from build123d import *

# Parameters (mm, degrees)
SKETCH1_R           = 45.5
SKETCH1_R_2         = 29.5
BOSS_EXTRUDE1_DEPTH = 4
SKETCH2_R           = 37.5
SKETCH2_R_2         = 29.5
BOSS_EXTRUDE2_DEPTH = 79.3
SKETCH4_R           = 1.55
CUT_EXTRUDE1_DEPTH  = 83.3
CIRPATTERN1_COUNT   = 3
SKETCH6_R           = 2
CUT_EXTRUDE2_DEPTH  = 6
CIRPATTERN2_COUNT   = 3
SKETCH8_R           = 30.5
CUT_EXTRUDE4_DEPTH  = 6


with BuildPart() as part:
    # Sketch1 → Boss-Extrude1 (new body)
    with BuildSketch(Plane(origin=(0, 0, 0), x_dir=(1, 0, 0), z_dir=(0, 1, 0))):
        with Locations(Location((0, 0, 0), (0, 0, 270))):
            Circle(SKETCH1_R)
        with Locations(Location((0, 0, 0), (0, 0, 270))):
            Circle(SKETCH1_R_2, mode=Mode.SUBTRACT)
    extrude(amount=BOSS_EXTRUDE1_DEPTH)

    # Sketch2 → Boss-Extrude2 (add)
    with BuildSketch(Plane(origin=(0, 4, 0), x_dir=(1, 0, 0), z_dir=(0, 1, 0))):
        with Locations(Location((0, 0, 0), (0, 0, 270))):
            Circle(SKETCH2_R)
        with Locations(Location((0, 0, 0), (0, 0, 270))):
            Circle(SKETCH2_R_2, mode=Mode.SUBTRACT)
    extrude(amount=BOSS_EXTRUDE2_DEPTH)

    # Sketch4 → Cut-Extrude1 (cut)
    with BuildSketch(Plane(origin=(0, 4, 0), x_dir=(1, 0, 0), z_dir=(0, 1, 0))):
        with Locations(Location((0, 41.5, 0), (0, 0, 270))):
            Circle(SKETCH4_R)
    cut_extrude1 = extrude(amount=-CUT_EXTRUDE1_DEPTH, mode=Mode.SUBTRACT)

    # CirPattern1: Cut-Extrude1 ×3 about axis
    cirpattern1_axis = Axis((0, 0, 0), (0, 1, 0))
    for i in range(1, CIRPATTERN1_COUNT):
        add(cut_extrude1.rotate(cirpattern1_axis, i * 360 / CIRPATTERN1_COUNT), mode=Mode.SUBTRACT)

    # Sketch6 → Cut-Extrude2 (cut)
    with BuildSketch(Plane(origin=(0, 83.3, 0), x_dir=(1, 0, 0), z_dir=(0, 1, 0))):
        with Locations(Location((-29.011851027, 16.75, 0), (0, 0, 270))):
            Circle(SKETCH6_R)
    cut_extrude2 = extrude(amount=-CUT_EXTRUDE2_DEPTH, mode=Mode.SUBTRACT)

    # CirPattern2: Cut-Extrude2 ×3 about axis
    cirpattern2_axis = Axis((0, 0, 0), (0, 1, 0))
    for i in range(1, CIRPATTERN2_COUNT):
        add(cut_extrude2.rotate(cirpattern2_axis, i * 360 / CIRPATTERN2_COUNT), mode=Mode.SUBTRACT)

    # Sketch8 → Cut-Extrude4 (cut)
    with BuildSketch(Plane.XZ):
        with Locations(Location((0, 0, 0), (0, 0, 270))):
            Circle(SKETCH8_R)
    extrude(amount=-CUT_EXTRUDE4_DEPTH, mode=Mode.SUBTRACT)


solid = part.part
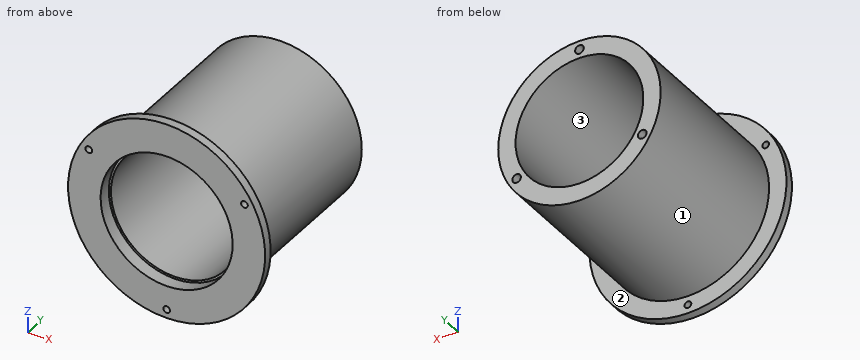
Model file for the job. Use its own axes, mm. Face numbers are marked on the shaded views. Coordinates: 2 decimals unless noted, no trailing zeros. Write each loop counter-clockwise with the first axis right and the second up, starting at its lowest first coordinate (ties: lowest second). Pieces come first, ordered by that corner, then holes. Notation, with made-up numbers: (-39.75, 2) -> (0.25, 2) arc R18 ccw to (0.25, 24) -> close; hole circle Ø8 at (56, -19). An arc over 180 degrees is marked (long way). One line per item, written item: value. Start each with the question number.
1) Slice it at A-A on z = 0. Write the cut outline in (x, y).
2) Flat gauge pins, fed straight in: pin 1 Ø4 at (x, y) = (16.5, 28.5) entering from -Z; pin 2 Ø6.5 at (x, z) = (-29.01, -16.75) entering from -Y; pin 3 Ø5 at (y, z) = (56, 14) entering from -X; pin 4 Ø3 at (x, z) = (-35.94, 20.75) entering from -Y. Where does each tip first touch, or does it go through?
3) Slice it at C-C on x = -14. Write the cut outline in (y, z), then the cut area to 3 significant figures.
4) Slice it at B-B on x = 0. Write the cut outline in (y, z).
5) Slice it at D-D on y = 37.5. Write the cut outline in (x, z).
6) Probe probe 1 along X at (y, z) = (53, 0); probe 2 along X at (y, z) = (20, -9.5); probe 3 along X at (y, z) = (81.85, -16.75). List the from-to ranges inside material, lowest first.
7) Pull direction X, two halves, no side cores. Call the marked faces 1, 2 and 3: +X half, -X half, draft (parallel to the pull), parting line (faces both ways), or undercut.
Answers follow:
1. outline: (-45.5, 0) -> (-30.5, 0) -> (-30.5, 6) -> (-29.5, 6) -> (-29.5, 83.3) -> (-37.5, 83.3) -> (-37.5, 4) -> (-45.5, 4) -> close; (29.5, 6) -> (30.5, 6) -> (30.5, 0) -> (45.5, 0) -> (45.5, 4) -> (37.5, 4) -> (37.5, 83.3) -> (29.5, 83.3) -> close
2. pin 1: z = -34.58
2. pin 2: y = 0
2. pin 3: x = -35.69
2. pin 4: through
3. outline: (0, -43.29) -> (4, -43.29) -> (4, -34.79) -> (83.3, -34.79) -> (83.3, -25.97) -> (6, -25.97) -> (6, -27.1) -> (0, -27.1) -> close; (0, 27.1) -> (6, 27.1) -> (6, 25.97) -> (83.3, 25.97) -> (83.3, 34.79) -> (4, 34.79) -> (4, 43.29) -> (0, 43.29) -> close
3. area: 1,520 mm2
4. outline: (0, -45.5) -> (4, -45.5) -> (4, -43.05) -> (0, -43.05) -> close; (0, -39.95) -> (4, -39.95) -> (4, -37.5) -> (83.3, -37.5) -> (83.3, -29.5) -> (6, -29.5) -> (6, -30.5) -> (0, -30.5) -> close; (0, 30.5) -> (6, 30.5) -> (6, 29.5) -> (83.3, 29.5) -> (83.3, 31.5) -> (77.3, 31.5) -> (77.3, 35.5) -> (83.3, 35.5) -> (83.3, 37.5) -> (4, 37.5) -> (4, 45.5) -> (0, 45.5) -> close
5. outline: circle Ø75 at (0, 0); hole circle Ø59 at (0, 0)
6. probe 1: -37.5 to -29.5, 29.5 to 37.5
6. probe 2: -36.28 to -27.93, 27.93 to 36.28
6. probe 3: -33.55 to -31.01, -27.01 to -24.28, 24.28 to 27.01, 31.01 to 33.55
7. face 1: parting line
7. face 2: draft
7. face 3: undercut
